Check sheet for the modelled part. Datum: model origin and axes. Units: mm. A direction names the side the tool comes from. Coordinates: 2 decimals unless noted, no trailing zeros. Write each loop counter-clockwise with the first axis right and the second up, starting at its lowest first coordinate (ties: lowest second). Pieces come first, ordered by that corner, then holes. Notation, with made-up numbers: (-1, -33) -> (36, -33) arc R29 cw to (36, -6) -> close; hole circle Ø11 at (80.25, 81.25). An arc over 180 degrees is marked (long way). Put each result on its own line as item: value.
```python
from build123d import *

# Parameters (mm, degrees)
EXTRUDE_1_DEPTH     = 3
SKETCH_2_W          = 5
SKETCH_2_H          = 3
CUT_EXTRUDE_1_DEPTH = 176
SKETCH_3_W          = 146.2
SKETCH_3_H          = 3
EXTRUDE_2_DEPTH     = 5
SKETCH_4_R          = 1.7
CUT_EXTRUDE_2_DEPTH = 5
CUT_EXTRUDE_3_DEPTH = 10
FILLET_1_R          = 5
SKETCH_7_W          = 146.2
SKETCH_7_H          = 3
EXTRUDE_3_DEPTH     = 20
SKETCH_8_R          = 3.2
CUT_EXTRUDE_4_DEPTH = 20
SKETCH_9_R          = 1.2
CUT_EXTRUDE_5_DEPTH = 20
FILLET_2_R          = 10
SKETCH_10_R         = 1.7
CUT_EXTRUDE_6_DEPTH = 3


with BuildPart() as part:
    # 草图1 → 凸台-拉伸1 (new body)
    with BuildSketch(Plane(origin=(0, 0, 0), x_dir=(1, 0, 0), z_dir=(0, 1, 0))):
        Polygon((-25, -73.1), (-25, -76.1), (-20, -76.1), (-20, -73.1), (-13.7, -73.1), (-13.7, -68.1), (-15.4, -68.1), (-15.4, -65.1), (-13.7, -65.1), (-13.7, -60.1), (-10.3, -60.1), (-10.3, -65.1), (-8.6, -65.1), (-8.6, -68.1), (-10.3, -68.1), (-10.3, -73.1), (-4, -73.1), (-4, -76.1), (4, -76.1), (4, -73.1), (10.3, -73.1), (10.3, -68.1), (8.6, -68.1), (8.6, -65.1), (10.3, -65.1), (10.3, -60.1), (13.7, -60.1), (13.7, -65.1), (15.4, -65.1), (15.4, -68.1), (13.7, -68.1), (13.7, -73.1), (20, -73.1), (20, -76.1), (25, -76.1), (25, -73.1), (35, -73.1), (35, 73.1), (25, 73.1), (25, 76.1), (20, 76.1), (20, 73.1), (13.7, 73.1), (13.7, 68.1), (15.4, 68.1), (15.4, 65.1), (13.7, 65.1), (13.7, 60.1), (10.3, 60.1), (10.3, 65.1), (8.6, 65.1), (8.6, 68.1), (10.3, 68.1), (10.3, 73.1), (4, 73.1), (4, 76.1), (-4, 76.1), (-4, 73.1), (-10.3, 73.1), (-10.3, 68.1), (-8.6, 68.1), (-8.6, 65.1), (-10.3, 65.1), (-10.3, 60.1), (-13.7, 60.1), (-13.7, 65.1), (-15.4, 65.1), (-15.4, 68.1), (-13.7, 68.1), (-13.7, 73.1), (-20, 73.1), (-20, 76.1), (-25, 76.1), (-25, 73.1), (-35, 73.1), (-35, -73.1), align=None)
    extrude(amount=EXTRUDE_1_DEPTH)

    # 草图2 → 切除-拉伸1 (cut)
    with BuildSketch(Plane.XY.offset(73.1)):
        with Locations((-32.5, 1.5)):
            Rectangle(SKETCH_2_W, SKETCH_2_H)
    extrude(amount=-CUT_EXTRUDE_1_DEPTH, mode=Mode.SUBTRACT)

    # 草图3 → 凸台-拉伸2 (add)
    with BuildSketch(Plane(origin=(35, 0, 0), x_dir=(0, 0, -1), z_dir=(1, 0, 0))):
        with Locations((0, 1.5)):
            Rectangle(SKETCH_3_W, SKETCH_3_H)
    extrude(amount=EXTRUDE_2_DEPTH)

    # 草图4 → 切除-拉伸2 (cut)
    with BuildSketch(Plane(origin=(0, 3, 0), x_dir=(1, 0, 0), z_dir=(0, 1, 0))):
        with Locations(Location((-19.75, -58.1, 0), (0, 0, 270))):
            Circle(SKETCH_4_R)
        with Locations(Location((19.25, -58.1, 0), (0, 0, 270))):
            Circle(SKETCH_4_R)
        with Locations(Location((19.25, 58.1, 0), (0, 0, 270))):
            Circle(SKETCH_4_R)
        with Locations(Location((-19.75, 58.1, 0), (0, 0, 270))):
            Circle(SKETCH_4_R)
    extrude(amount=-CUT_EXTRUDE_2_DEPTH, mode=Mode.SUBTRACT)

    # 草图5 → 切除-拉伸3 (cut)
    with BuildSketch(Plane(origin=(0, 3, 0), x_dir=(1, 0, 0), z_dir=(0, 1, 0))):
        Polygon((-30, -56.331395183), (-14.5, -43.1), (0, -43.1), (22, -43.1), (22, 43.1), (-14.5, 43.1), (-30, 56.331395183), align=None)
    extrude(amount=-CUT_EXTRUDE_3_DEPTH, mode=Mode.SUBTRACT)

    # 圆角1
    fillet_1_edges = [part.edges().sort_by_distance(p)[0] for p in [
        (-30, 1.5, 56.331395183),
        (-30, 1.5, -56.331395183),
        (-14.5, 1.5, -43.1),
        (22, 1.5, -43.1),
        (22, 1.5, 43.1),
        (-14.5, 1.5, 43.1),
    ]]
    fillet(fillet_1_edges, radius=FILLET_1_R)

    # 草图7 → 凸台-拉伸3 (add)
    with BuildSketch(Plane(origin=(40, 0, 0), x_dir=(0, 0, -1), z_dir=(1, 0, 0))):
        with Locations((0, 1.5)):
            Rectangle(SKETCH_7_W, SKETCH_7_H)
    extrude(amount=EXTRUDE_3_DEPTH)

    # 草图8 → 切除-拉伸4 (cut)
    with BuildSketch(Plane(origin=(0, 3, 0), x_dir=(1, 0, 0), z_dir=(0, 1, 0))):
        with Locations(Location((47, -2, 0), (0, 0, 270))):
            Circle(SKETCH_8_R)
    extrude(amount=-CUT_EXTRUDE_4_DEPTH, mode=Mode.SUBTRACT)

    # 草图9 → 切除-拉伸5 (cut)
    with BuildSketch(Plane(origin=(0, 3, 0), x_dir=(1, 0, 0), z_dir=(0, 1, 0))):
        with Locations(Location((37, -2, 0), (0, 0, 270))):
            Circle(SKETCH_9_R)
        with BuildLine():
            Line((35.8, 13), (35.8, 28))
            ThreePointArc((35.8, 28), (37, 29.2), (38.2, 28))
            Line((38.2, 28), (38.2, 13))
            ThreePointArc((38.2, 13), (37, 11.8), (35.8, 13))
        make_face()
        with BuildLine():
            Line((38.2, -17), (38.2, -32))
            ThreePointArc((38.2, -32), (37, -33.2), (35.8, -32))
            Line((35.8, -32), (35.8, -17))
            ThreePointArc((35.8, -17), (37, -15.8), (38.2, -17))
        make_face()
    extrude(amount=-CUT_EXTRUDE_5_DEPTH, mode=Mode.SUBTRACT)

    # 圆角2
    fillet_2_edges = [part.edges().sort_by_distance(p)[0] for p in [
        (60, 1.5, 73.1),
        (60, 1.5, -73.1),
    ]]
    fillet(fillet_2_edges, radius=FILLET_2_R)

    # 草图10 → 切除-拉伸6 (cut)
    with BuildSketch(Plane(origin=(0, 3, 0), x_dir=(1, 0, 0), z_dir=(0, 1, 0))):
        with Locations(Location((26, -27, 0), (0, 0, 270))):
            Circle(SKETCH_10_R)
        with Locations(Location((26, 23, 0), (0, 0, 270))):
            Circle(SKETCH_10_R)
        with Locations(Location((26, 0, 0), (0, 0, 270))):
            Circle(SKETCH_10_R)
    extrude(amount=-CUT_EXTRUDE_6_DEPTH, mode=Mode.SUBTRACT)


solid = part.part
```
Q1. Cross-section at A-A (x = 6). Record the cut outline in (y, z).
Recorded:
outline: (0, -73.1) -> (3, -73.1) -> (3, -43.1) -> (0, -43.1) -> close; (0, 43.1) -> (3, 43.1) -> (3, 73.1) -> (0, 73.1) -> close
Q2. Cross-section at C-C (y = 1.55). State how many separate pieces and enclosed holes the cut face has, plus the area to 3 significant figures.
Recorded:
separate pieces: 1
enclosed holes: 11
area: 8,150 mm2
Q3. Tool access check on faces 1 (the flat face through (0, 1, -76.1)), 2 (the flat face through (7, 1, 73.1)), 3 (the flat face through (24, 3, 1)), 4 (the flat face through (17, 1, -73.1)), 5 (the cylindrical face through (-14.409, 1.479, 43.417)). Record the directions out of +Z, -Z, +X, -X, +Y, -Y that give a thin tool (end or side, any length) a straight path to the whole face; none if there is none.
Recorded:
face 1: -Z, +X, -X, +Y, -Y
face 2: +Z, +Y, -Y
face 3: +Z, -Z, +X, -X, +Y
face 4: -Z, +Y, -Y
face 5: -X, +Y, -Y
Q4. Depth check by flat-ended pin: P1, Ø0.9, axis at x = 12, y = 1.5, coming from the -Z side; P2, Ø0.5, axis at x = 14.5, y = 1, coming from the +Z side; P3, Ø0.9, axis at x = 41.5, y = 2, coming from the -Z side; P4, Ø10, axis at x = -20.5, z = -36, coming from the +Y side. Enter the tip coordinate at first touch or a pass-through.
Recorded:
P1: stops at z = -60.1
P2: stops at z = 73.1
P3: stops at z = -73.1
P4: passes through
Q5. Cross-section at D-D (z = -7). Record the cut outline in (x, y), plus the area to 3 significant figures.
Recorded:
outline: (22, 0) -> (60, 0) -> (60, 3) -> (22, 3) -> close
area: 114 mm2
Q6. Cross-section at B-B (z = 27). Record the cut outline in (x, y).
Recorded:
outline: (22, 0) -> (24.3, 0) -> (24.3, 3) -> (22, 3) -> close; (27.7, 0) -> (35.8, 0) -> (35.8, 3) -> (27.7, 3) -> close; (38.2, 0) -> (60, 0) -> (60, 3) -> (38.2, 3) -> close
Q7. Material ranges on line 1 along Z through (x, y) = (9, 2); line 2 along X through (y, z) = (0.3, 65); line 3 along X through (y, z) = (0.8, -58.1), recorded low to high.
Recorded:
line 1: z = -73.1 to -68.1, -65.1 to -43.1, 43.1 to 65.1, 68.1 to 73.1
line 2: x = -30 to -13.7, -10.3 to 10.3, 13.7 to 59.82
line 3: x = -29.97 to -21.45, -18.05 to 17.55, 20.95 to 60
Q8. Mould release check, pull along X, two halves, no side actions. Record for faces 6 (the flat face through (22, 2, 1)), 7 (the flat face through (-10.3, 1, 71)), 8 (the flat face through (-23, 1, 76.1)): released by +X, released by -X, zero draft, split by the parting line, or undercut.
Recorded:
face 6: released by -X
face 7: undercut
face 8: zero draft
